Work out the finished part from the listing and answer in its coordinate system (mm). A direction names the side the tool comes from. Give positions to 0.01 mm unless a question says otherwise; leave off trailing zeros. Loops run counter-clockwise (first coordinate to the right, second up) from the corner with the lowest first, then second, coordinate; pieces in that order, holes last. Notation, with made-up numbers: (13.25, 21) - (31.25, 21) arc R26 ccw to (31.25, 49) - close; hole circle Ø6 at (2.25, 33). An arc over 180 degrees is marked (long way). One line per question, with ' | ' between items.
Autodesk Inventor part; units mm, degrees
ref_plane "YZ Plane" through (0, 0, 0) normal (1, 0, 0) x (0, 1, 0)
ref_plane "XZ Plane" through (0, 0, 0) normal (0, 1, 0) x (-1, 0, 0)
ref_plane "XY Plane" through (0, 0, 0) normal (0, 0, 1) x (1, 0, 0)
sketch "スケッチ1" plane through (0, 0, 0) normal (0, 0, 1) x (1, 0, 0)
  circle A0 centre (0, 0) radius 2.5
  dimension "d0" = 5
extrude "押し出し1" add sketch "スケッチ1" along normal blind 104
sketch "スケッチ2" plane through (0, 0, 104) normal (0, 0, 1) x (1, 0, 0)
  line L0 (4.6188, 0) -> (2.3094, -4)
  line L1 (2.3094, -4) -> (-2.3094, -4)
  line L2 (-2.3094, -4) -> (-4.6188, 0)
  line L3 (-4.6188, 0) -> (-2.3094, 4)
  line L4 (-2.3094, 4) -> (2.3094, 4)
  line L5 (2.3094, 4) -> (4.6188, 0)
  point P0 (0, 0)
  point P1 (0, 0)
  dimension "d3" = 8
extrude "押し出し2" add sketch "スケッチ2" along normal blind 3.5
sketch "スケッチ3" plane through (0, 0, 107.5) normal (0, 0, 1) x (1, 0, 0)
  circle A0 centre (0, 0) radius 2.5
  dimension "d6" = 5
extrude "押し出し3" add sketch "スケッチ3" along normal blind 12.5
properties part number "aircylinder16_100_part2_sa" material "アルミニウム 6061-AHC"
1. Flat-ended cylindrical pins translate along their axes: pin 1 (1 mm diameter, centred on x = -2, z = 86.5, fed in from -Y); pin 2 (1.5 mm diameter, centred on x = -2.5, y = 1, fed in from -Z); pin 3 (4 mm diameter, centred on y = 0.5, z = 18, fed in from -X); pin 4 (3 mm diameter, centred on x = 3.5, z = 79.5, fed in from +Y). Find the tip coordinate at first contact, or state that the pin passes through.
Evaluation:
pin 1: y = -2 | pin 2: z = 0 | pin 3: x = -2.5 | pin 4: y = 1.5
2. Which of the six approach directions +Z, -Z, +X, -X, +Y, -Y give full straight-line access (tool end or side, diameter ignored) to faces 1 (the flat face through (-3.448, -2.028, 105.726)), 2 (the flat face through (2, 2, 107.5)), 3 (the flat face through (2, 2, 104))?
Evaluation:
face 1: +Z, -Z, -X, -Y | face 2: +Z | face 3: -Z
3. Find section C-C on z = 65. Write down the section's boundary in (x, y).
Evaluation:
outline: circle Ø5 at (0, 0)
4. Find section B-B on y = 1. Write down the section's boundary in (x, z).
Evaluation:
outline: (-4.04, 104) - (-2.29, 104) - (-2.29, 0) - (2.29, 0) - (2.29, 104) - (4.04, 104) - (4.04, 107.5) - (2.29, 107.5) - (2.29, 120) - (-2.29, 120) - (-2.29, 107.5) - (-4.04, 107.5) - close
5. Consider L1, parallel to Y at x = -0.25, z = 78; L2, parallel to Z at x = 3.5, y = -1.25; L3, parallel to X at y = -1, z = 40.5. Determine where each line is inside the solid, lowest interval first.
Evaluation:
L1: -2.49 to 2.49 | L2: 104 to 107.5 | L3: -2.29 to 2.29
6. Find section A-A on x = 0. Write down the section's boundary in (y, z).
Evaluation:
outline: (-4, 104) - (-2.5, 104) - (-2.5, 0) - (2.5, 0) - (2.5, 104) - (4, 104) - (4, 107.5) - (2.5, 107.5) - (2.5, 120) - (-2.5, 120) - (-2.5, 107.5) - (-4, 107.5) - close
